Build history of the part. All positions in model axes, mm. Face numbers are marked on the shaded views. Round coordinates to 2 decimals unless told otherwise and drop trailing zeros. Write each loop counter-clockwise with the first axis right and the second up, starting at its lowest first coordinate (ties: lowest second). Pieces come first, ordered by that corner, then holes. Notation, with made-up numbers: M -37,22.25 L -25,22.25 A17 cw -25,53.25 Z; hole C 74.5,16 d8. An arc over 180 degrees is marked long. Use a Markdown table: item, result.
from build123d import *

# Parameters (mm, degrees)
ESBO_O1_R                = 2.1
ESBO_O1_R_2              = 14
RESSALTO_EXTRUS_O1_DEPTH = 3
FILETE1_R                = 5


with BuildPart() as part:
    # Esboço1 → Ressalto-extrusão1 (new body)
    with BuildSketch(Plane.XY):
        with BuildLine():
            Line((-14.662878299, -19), (14.662878299, -19))
            ThreePointArc((14.662878299, -19), (21.539603979, -10.585152829), (24, 0))
            ThreePointArc((24, 0), (-10.585152829, 21.539603979), (-14.662878299, -19))
        make_face()
        with Locations((-20, 0)):
            Circle(ESBO_O1_R, mode=Mode.SUBTRACT)
        Circle(ESBO_O1_R_2, mode=Mode.SUBTRACT)
        with Locations((20, 0)):
            Circle(ESBO_O1_R, mode=Mode.SUBTRACT)
    extrude(amount=RESSALTO_EXTRUS_O1_DEPTH)

    # Filete1
    filete1_edges = [part.edges().sort_by_distance(p)[0] for p in [
        (-14.662878299, -19, 1.5),
        (14.662878299, -19, 1.5),
    ]]
    fillet(filete1_edges, radius=FILETE1_R)


solid = part.part
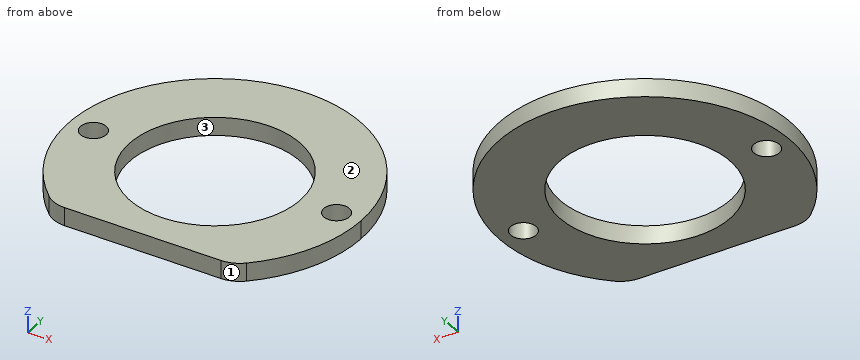
Q1. Cut at B-B on x = 0. Give the cut face in (y, z).
Response values:
| item | result |
|---|---|
| outline | M -19,0 L -14,0 L -14,3 L -19,3 Z; M 14,0 L 24,0 L 24,3 L 14,3 Z |
Q2. Drop flat-ended pins along their axis: P1, Ø1, axis at x = -17.5, z = 2.5, coming from the -Y side; P2, Ø6.5, axis at x = 20, y = 0, coming from the +Z side; P3, Ø17, axis at x = 0, y = 0, coming from the -Z side; P4, Ø1.5, axis at x = 2, z = 0.5, coming from the +Y side. Give the stop position or say it passes through.
Response values:
| item | result |
|---|---|
| P1 | stops at y = -16.94 |
| P2 | stops at z = 3 |
| P3 | passes through |
| P4 | stops at y = 23.97 |
Q3. Drill centre lines: L1, parallel to Y at x = 0, z = 0.4; L2, parallel to X at y = -9, z = 1.4; L3, parallel to Y at x = -20, z = 0.75. Where is each one in solid material? Low to high.
Response values:
| item | result |
|---|---|
| L1 | y = -19 to -14, 14 to 24 |
| L2 | x = -22.25 to -10.72, 10.72 to 22.25 |
| L3 | y = -13.27 to -2.1, 2.1 to 13.27 |
Q4. Cut at C-C on y = -7. Give the cut face in (x, z), and give its area (3 significant figures).
Response values:
| item | result |
|---|---|
| outline | M -22.96,0 L -12.12,0 L -12.12,3 L -22.96,3 Z; M 12.12,0 L 22.96,0 L 22.96,3 L 12.12,3 Z |
| area | 65.0 mm2 |
Q5. Two-plate mould, pull along Y, no slides. Class the marked faces 1, 2 and 3: +Y half, -Y half, draft (parallel to the pull), parting line (faces both ways), or undercut.
Response values:
| item | result |
|---|---|
| face 1 | -Y half |
| face 2 | draft |
| face 3 | undercut |
Q6. Cut at A-A on z = 1.55. Give the cut face in (x, y), and give its area (3 significant figures).
Response values:
| item | result |
|---|---|
| outline | M -16.23,-17.68 A5 ccw -12.85,-19 L 12.85,-19 A5 ccw 16.23,-17.68 A24 ccw long Z; hole C -20,0 d4.2; hole C 0,0 d28; hole C 20,0 d4.2 |
| area | 1,070 mm2 |
Q7. Cut at D-D on y = 1. Give the cut face in (x, z), and give its area (3 significant figures).
Response values:
| item | result |
|---|---|
| outline | M -23.98,0 L -21.85,0 L -21.85,3 L -23.98,3 Z; M -18.15,0 L -13.96,0 L -13.96,3 L -18.15,3 Z; M 13.96,0 L 18.15,0 L 18.15,3 L 13.96,3 Z; M 21.85,0 L 23.98,0 L 23.98,3 L 21.85,3 Z |
| area | 37.9 mm2 |
